Source: CAD feature listing. Evaluate the final solid. Frame: model axes, mm. Give positions to 0.01 mm unless a question says otherwise; leave off trailing zeros. Write each loop counter-clockwise with the first axis right and the second up, starting at its lowest first coordinate (ties: lowest second). Pieces come first, ordered by that corner, then holes.
```python
from build123d import *

# Parameters (mm, degrees)
F0_R     = 16.15
F0_R_2   = 11
F1_DEPTH = 10
F2_SIZE  = 0.3
F3_SIZE  = 0.5


with BuildPart() as f1:
    # F0 (on Top) → F1 (new body)
    with BuildSketch(Plane.XY):
        Circle(F0_R)
        Circle(F0_R_2, mode=Mode.SUBTRACT)
    extrude(amount=F1_DEPTH)

    # F2
    f2_edges = [f1.edges().sort_by_distance(p)[0] for p in [
        (-11, 0, 10),
        (-11, 0, 0),
    ]]
    chamfer(f2_edges, length=F2_SIZE)

    # F3
    f3_edges = [f1.edges().sort_by_distance(p)[0] for p in [
        (-16.15, 0, 10),
        (-16.15, 0, 0),
    ]]
    chamfer(f3_edges, length=F3_SIZE)


solid = f1.part
```
1. Section query A-A (y = 0). Return loops of the section in (x, z).
2. Line query: probe 1 along Y at (x, z) = (0, 6.5); probe 2 along Y at (x, z) = (7, 4.75); probe 3 along X at (y, z) = (-6, 1). Output: solid intervals per line, ascending.
3. Section query C-C (z = 2.5). Return loops of the section in (x, y).
4. Pull-direction query (Y, two-part tool) for faces 1 (the flat face through (8, 8.2, 0)), 2 (the cylindrical face through (-3.501, -15.766, 4.937)), 3 (the cylindrical face through (-2.38, -10.74, 4.93)); classes: pulls with the +Y half, pulls with the -Y half, needs draft (parallel to the pull), parting line crosses it, or undercut.
5. Pin query (flat end, axial travel): P1, Ø5, axis at y = 11, z = 6, coming from the -X side; P2, Ø4, axis at y = -9, z = 2.5, coming from the +X side; P3, Ø1.5, axis at x = 4, z = 4.5, coming from the -Y side. Return the tip coordinate at first contact, or that it passes through.
The answers:
1. outline: (-16.15, 0.5) - (-15.65, 0) - (-11.3, 0) - (-11, 0.3) - (-11, 9.7) - (-11.3, 10) - (-15.65, 10) - (-16.15, 9.5) - close; (11, 0.3) - (11.3, 0) - (15.65, 0) - (16.15, 0.5) - (16.15, 9.5) - (15.65, 10) - (11.3, 10) - (11, 9.7) - close
2. probe 1: y = -16.15 to -11, 11 to 16.15
2. probe 2: y = -14.55 to -8.49, 8.49 to 14.55
2. probe 3: x = -14.99 to -9.22, 9.22 to 14.99
3. outline: circle Ø32.3 at (0, 0); hole circle Ø22 at (0, 0)
4. face 1: needs draft
4. face 2: parting line crosses it
4. face 3: undercut
5. P1: stops at x = -13.73
5. P2: stops at x = 14.55
5. P3: stops at y = -15.82
